```python
from build123d import *

# Parameters (mm, degrees)
SKETCH1_R           = 3.2
SKETCH1_R_2         = 2.929016319
BOSS_EXTRUDE1_DEPTH = 2.2
SKETCH2_R           = 3.2
SKETCH2_R_2         = 1.3
BOSS_EXTRUDE2_DEPTH = 15.2
SKETCH3_R           = 3.2
BOSS_EXTRUDE3_DEPTH = 1.9
SKETCH4_R           = 1.3
BOSS_EXTRUDE4_DEPTH = 0.2


with BuildPart() as part:
    # Sketch1 → Boss-Extrude1 (new body)
    with BuildSketch(Plane.XY):
        with Locations((-32.2, 44.45)):
            Circle(SKETCH1_R)
        with Locations((-32.2, 44.45)):
            Circle(SKETCH1_R_2, mode=Mode.SUBTRACT)
    extrude(amount=BOSS_EXTRUDE1_DEPTH)

    # Sketch2 → Boss-Extrude2 (add)
    with BuildSketch(Plane.XY.offset(2.2)):
        with Locations((-32.2, 44.45)):
            Circle(SKETCH2_R)
        with Locations((-32.2, 44.45)):
            Circle(SKETCH2_R_2, mode=Mode.SUBTRACT)
    extrude(amount=BOSS_EXTRUDE2_DEPTH)

    # Sketch3 → Boss-Extrude3 (add)
    with BuildSketch(Plane.XY.offset(17.4)):
        with Locations((-32.2, 44.45)):
            Circle(SKETCH3_R)
        Polygon((-34.75, 42.977756814), (-32.2, 41.505513627), (-29.65, 42.977756814), (-29.65, 45.922243186), (-32.2, 47.394486373), (-34.75, 45.922243186), align=None, mode=Mode.SUBTRACT)
    extrude(amount=BOSS_EXTRUDE3_DEPTH)

    # Sketch4 → Boss-Extrude4 (add)
    with BuildSketch(Plane(origin=(0, 0, 2.2), x_dir=(-1, 0, 0), z_dir=(0, 0, -1))):
        with Locations((32.2, 44.45)):
            Circle(SKETCH4_R)
    extrude(amount=-BOSS_EXTRUDE4_DEPTH)


solid = part.part
```
Verification items for the finished model (mm, model axes). A direction names the side the tool comes from. Round coordinates to 2 decimals unless told otherwise and drop trailing zeros. Order: outer loops, then holes, each group sorted by start corner. A loop starts at its lowest first (then second) coordinate and runs counter-clockwise, first axis right, second up. Notation, with made-up numbers: (49.25, 12) -> (90.25, 12) arc R19 ccw to (90.25, 41) -> close; hole circle Ø8 at (-5.5, 67.25). An arc over 180 degrees is marked (long way). Put each result on its own line as item: value. Start each with the question number.
(1) Section check D-D (x = -30.5). Enter the section's corners in (y, z).
(2) Tool access check on faces 1 (the face through (-30.91, 46.65, 18.34)), 2 (the face through (-34.36, 46.43, 1.08)). Record the directions out of +Z, -Z, +X, -X, +Y, -Y that give a thin tool (end or side, any length) a straight path to the whole face; none if there is none.
(3) Draft check along Y on faces 3 (the face through (-31, 47, 19.3)), 4 (the face through (-33, 43, 17.4)), 5 (the face through (-31.501, 45.546, 9.795)), 6 (the face through (-29.148, 45.411, 9.515)). Enter one of: +Y half, -Y half, draft (parallel to the pull), parting line (faces both ways), or undercut.
(4) Section check C-C (x = -33). Enter the section's corners in (y, z), then the cut area to 3 significant figures.
(5) Section check A-A (z = 18). Enter the section's corners in (x, y), then the cut area to 3 significant figures.
(6) Depth check by flat-ended pin: pin 1 Ø3.5 at (x, y) = (-32.2, 44.45) entering from -Z; pin 2 Ø1 at (x, z) = (-30.5, 12.5) entering from -Y; pin 3 Ø3 at (x, y) = (-32.5, 44.5) entering from +Z. Enter the tip coordinate at first touch or a pass-through.
(7) Material ranges on line 1 along Y through (x, z) = (-32.2, 1.7); line 2 along Y through (x, z) = (-32.2, 14); line 3 along Z through (x, y) = (-31.25, 46.25), recorded low to high.
(8) Section check B-B (y = 44.45). Enter the section's corners in (x, z), then the cut area to 3 significant figures.
Completed:
1. outline: (41.74, 0) -> (42.06, 0) -> (42.06, 2.2) -> (46.84, 2.2) -> (46.84, 0) -> (47.16, 0) -> (47.16, 19.3) -> (46.41, 19.3) -> (46.41, 17.4) -> (42.49, 17.4) -> (42.49, 19.3) -> (41.74, 19.3) -> close
2. face 1: +Z
2. face 2: -Z
3. face 3: draft
3. face 4: undercut
3. face 5: undercut
3. face 6: parting line
4. outline: (41.35, 0) -> (41.63, 0) -> (41.63, 2.2) -> (47.27, 2.2) -> (47.27, 0) -> (47.55, 0) -> (47.55, 19.3) -> (46.93, 19.3) -> (46.93, 17.4) -> (45.47, 17.4) -> (45.47, 2.4) -> (43.43, 2.4) -> (43.43, 17.4) -> (41.97, 17.4) -> (41.97, 19.3) -> (41.35, 19.3) -> close
4. area: 67.0 mm2
5. outline: circle Ø6.4 at (-32.2, 44.45); hole (-34.75, 42.98) -> (-32.2, 41.51) -> (-29.65, 42.98) -> (-29.65, 45.92) -> (-32.2, 47.39) -> (-34.75, 45.92) -> close
5. area: 9.64 mm2
6. pin 1: stops at z = 2.2
6. pin 2: stops at y = 41.48
6. pin 3: stops at z = 17.4
7. line 1: y = 41.25 to 41.52, 47.38 to 47.65
7. line 2: y = 41.25 to 43.15, 45.75 to 47.65
7. line 3: z = 2.2 to 17.4
8. outline: (-35.4, 0) -> (-35.13, 0) -> (-35.13, 2.2) -> (-29.27, 2.2) -> (-29.27, 0) -> (-29, 0) -> (-29, 19.3) -> (-29.65, 19.3) -> (-29.65, 17.4) -> (-30.9, 17.4) -> (-30.9, 2.4) -> (-33.5, 2.4) -> (-33.5, 17.4) -> (-34.75, 17.4) -> (-34.75, 19.3) -> (-35.4, 19.3) -> close
8. area: 61.9 mm2
